Can you work these out from the model? Positions are in its coordinate system, mm. A direction names the side the tool comes from. Coordinates: 2 decimals unless noted, no trailing zeros. Write each loop counter-clockwise with the first axis right and the second up, starting at its lowest first coordinate (ties: lowest second). Pieces come first, ordered by that corner, then holes.
```python
from build123d import *

# Parameters (mm, degrees)
SKETCH1_R           = 2
SKETCH1_R_2         = 1.95
SKETCH1_R_3         = 0.25
BOSS_EXTRUDE1_DEPTH = 5


with BuildPart() as part:
    # Sketch1 → Boss-Extrude1 (new body)
    with BuildSketch(Plane.XY):
        Polygon((-104.194627872, 87.590269756), (122.373914623, 87.590269756), (154.089643375, 55.874541003), (154.089643375, -85.694001492), (122.373914623, -117.409730244), (-104.194627872, -117.409730244), (-135.910356625, -85.694001492), (-135.910356625, 55.874541003), align=None)
        with Locations((121.614769641, 74.207279114)):
            Circle(SKETCH1_R, mode=Mode.SUBTRACT)
        with Locations((140.706652733, 55.115396022)):
            Circle(SKETCH1_R, mode=Mode.SUBTRACT)
        with Locations((-103.435482891, 74.207279114)):
            Circle(SKETCH1_R, mode=Mode.SUBTRACT)
        with Locations((-103.435482891, -104.026739602)):
            Circle(SKETCH1_R, mode=Mode.SUBTRACT)
        with Locations((-122.527365983, 55.115396022)):
            Circle(SKETCH1_R, mode=Mode.SUBTRACT)
        with Locations((-122.527365983, -84.93485651)):
            Circle(SKETCH1_R, mode=Mode.SUBTRACT)
        with Locations((121.614769641, -104.026739602)):
            Circle(SKETCH1_R, mode=Mode.SUBTRACT)
        with Locations((140.706652733, -84.93485651)):
            Circle(SKETCH1_R, mode=Mode.SUBTRACT)
        with Locations((29.089643375, 77.590269756)):
            Circle(SKETCH1_R, mode=Mode.SUBTRACT)
        with Locations((29.089643375, -107.409730244)):
            Circle(SKETCH1_R, mode=Mode.SUBTRACT)
        with Locations((-7.910356625, -107.409730244)):
            Circle(SKETCH1_R, mode=Mode.SUBTRACT)
        with Locations((-7.910356625, 77.590269756)):
            Circle(SKETCH1_R, mode=Mode.SUBTRACT)
        with Locations((-90.910356625, 77.590269756)):
            Circle(SKETCH1_R, mode=Mode.SUBTRACT)
        with Locations((109.089643375, -107.409730244)):
            Circle(SKETCH1_R, mode=Mode.SUBTRACT)
        with Locations((99.089643375, -107.409730244)):
            Circle(SKETCH1_R, mode=Mode.SUBTRACT)
        with Locations((-80.910356625, 77.590269756)):
            Circle(SKETCH1_R, mode=Mode.SUBTRACT)
        with Locations((-90.910356625, -107.409730244)):
            Circle(SKETCH1_R, mode=Mode.SUBTRACT)
        with Locations((-80.910356625, -107.409730244)):
            Circle(SKETCH1_R, mode=Mode.SUBTRACT)
        with Locations((99.089643375, 77.590269756)):
            Circle(SKETCH1_R, mode=Mode.SUBTRACT)
        with Locations((109.089643375, 77.590269756)):
            Circle(SKETCH1_R, mode=Mode.SUBTRACT)
        with Locations((69.089643375, 75.590269756)):
            Circle(SKETCH1_R_2, mode=Mode.SUBTRACT)
        with Locations((-50.910356625, 75.590269756)):
            Circle(SKETCH1_R_2, mode=Mode.SUBTRACT)
        with Locations((-50.910356625, -105.409730244)):
            Circle(SKETCH1_R_2, mode=Mode.SUBTRACT)
        with Locations((69.089643375, -105.409730244)):
            Circle(SKETCH1_R_2, mode=Mode.SUBTRACT)
        with Locations((144.089643375, -14.909730244)):
            Circle(SKETCH1_R_2, mode=Mode.SUBTRACT)
        with Locations((-125.910356625, -14.909730244)):
            Circle(SKETCH1_R_2, mode=Mode.SUBTRACT)
        with Locations((9.089643375, -14.909730244)):
            Circle(SKETCH1_R_3, mode=Mode.SUBTRACT)
        Polygon((134.089643375, 47.590269756), (134.089643375, -77.409730244), (114.089643375, -97.409730244), (114.089643375, 67.590269756), align=None, mode=Mode.SUBTRACT)
        Polygon((-115.910356625, 47.590269756), (-115.910356625, -77.409730244), (-95.910356625, -97.409730244), (-95.910356625, 67.590269756), align=None, mode=Mode.SUBTRACT)
    extrude(amount=BOSS_EXTRUDE1_DEPTH)


solid = part.part
```
1. I'm going to push flat-ended pins straight in: P1, Ø2, axis at x = 120, y = -89, coming from the -Z side; P2, Ø2, axis at y = 58, z = 3, coming from the +X side. Where does each tip first touch, or does it pass through?
2. Which directions (+Z, -Z, +X, -X, +Y, -Y) give clear straight access to the entire face, cutting with the end or side of a thin tool? Please do faces 1 (the face through (123.95, 57.73, 2.46)), 2 (the face through (138.01, 71.954, 2.465)).
3. If we section it at A-A, the plane y = -21: List the corners of the cut face in (x, z) for me.
4. If we section it at B-B, the plane z = 0.8: Count the separate pieces of the cut face and the enclosed holes in it, plus the area to 3 significant figures.
5. If I drill on L1, parallel to X at y = 13, z = 0.3; L2, parallel to X at y = 52.5, z = 1.85; L3, parallel to Y at x = 98.5, z = 1.25, over which ranges is the centre line in solid material (lowest first)?
6. We'd pull the mould along X, two halves only. Please class faces 3 (the face through (-105.8, 57.7, 2.5)), 4 (the face through (138.454, -101.33, 2.465)), 5 (the face through (11, -13, 5)): released by +X, released by -X, zero draft, split by the parting line, or undercut.
Answers:
1. P1: passes through
1. P2: stops at x = 152.96
2. face 1: +Z, -Z
2. face 2: +Z, -Z, +X, +Y
3. outline: (-135.91, 0) - (-115.91, 0) - (-115.91, 5) - (-135.91, 5) - close; (-95.91, 0) - (114.09, 0) - (114.09, 5) - (-95.91, 5) - close; (134.09, 0) - (154.09, 0) - (154.09, 5) - (134.09, 5) - close
4. separate pieces: 1
4. enclosed holes: 29
4. area: 51,300 mm2
5. L1: x = -135.91 to -115.91, -95.91 to 114.09, 134.09 to 154.09
5. L2: x = -135.91 to -111, -95.91 to 114.09, 129.18 to 154.09
5. L3: y = -117.41 to -109.32, -105.5 to 75.68, 79.5 to 87.59
6. face 3: undercut
6. face 4: released by +X
6. face 5: zero draft
